from build123d import *

# Parameters (mm, degrees)
CROQUIS1_W              = 10
CROQUIS1_H              = 60
CROQUIS1_R              = 2.5
SALIENTE_EXTRUIR1_DEPTH = 1.5
CROQUIS2_W              = 3
CROQUIS2_H              = 60
SALIENTE_EXTRUIR2_DEPTH = 12
CROQUIS4_R              = 32
CORTAR_EXTRUIR2_DEPTH   = 34.320414163
SKETCH1_W               = 13
SKETCH1_H               = 10
BOSS_EXTRUDE1_DEPTH     = 60
SKETCH2_R               = 2.5
CUT_EXTRUDE1_DEPTH      = 34.109666262
SKETCH3_W               = 10
SKETCH3_H               = 8.5
CUT_EXTRUDE2_DEPTH      = 62.613716005
SKETCH4_R               = 2
CUT_EXTRUDE3_DEPTH      = 34.648922717


with BuildPart() as part:
    # Croquis1 → Saliente-Extruir1 (new body)
    with BuildSketch(Plane(origin=(0, 0, 0), x_dir=(1, 0, 0), z_dir=(0, 1, 0))):
        Rectangle(CROQUIS1_W, CROQUIS1_H)
        with Locations(Location((0, 22.5, 0), (0, 0, 270))):
            Circle(CROQUIS1_R, mode=Mode.SUBTRACT)
        with Locations(Location((0, -22.5, 0), (0, 0, 270))):
            Circle(CROQUIS1_R, mode=Mode.SUBTRACT)
    extrude(amount=SALIENTE_EXTRUIR1_DEPTH)

    # Croquis2 → Saliente-Extruir2 (add)
    with BuildSketch(Plane(origin=(0, 1.5, 0), x_dir=(1, 0, 0), z_dir=(0, 1, 0))):
        with Locations((6.5, 0)):
            Rectangle(CROQUIS2_W, CROQUIS2_H)
    extrude(amount=-SALIENTE_EXTRUIR2_DEPTH)

    # Croquis4 → Cortar-Extruir2 (cut, through all)
    with BuildSketch(Plane.ZY.offset(-5)):
        with Locations((0, -38.5)):
            Circle(CROQUIS4_R)
    extrude(amount=-CORTAR_EXTRUIR2_DEPTH, mode=Mode.SUBTRACT)

    # Sketch1 → Boss-Extrude1 (add)
    with BuildSketch(Plane(origin=(0, 0, -30), x_dir=(-1, 0, 0), z_dir=(0, 0, -1))):
        with Locations((-1.5, 6.5)):
            Rectangle(SKETCH1_W, SKETCH1_H)
    extrude(amount=-BOSS_EXTRUDE1_DEPTH)

    # Sketch2 → Cut-Extrude1 (cut, through all)
    with BuildSketch(Plane.XZ):
        with Locations(Location((0, -22.5, 0), (0, 0, 270))):
            Circle(SKETCH2_R)
        with Locations(Location((0, 22.5, 0), (0, 0, 270))):
            Circle(SKETCH2_R)
    extrude(amount=-CUT_EXTRUDE1_DEPTH, mode=Mode.SUBTRACT)

    # Sketch3 → Cut-Extrude2 (cut, through all)
    with BuildSketch(Plane(origin=(0, 0, -30), x_dir=(-1, 0, 0), z_dir=(0, 0, -1))):
        with Locations((0, 4.25)):
            Rectangle(SKETCH3_W, SKETCH3_H)
    extrude(amount=-CUT_EXTRUDE2_DEPTH, mode=Mode.SUBTRACT)

    # Sketch4 → Cut-Extrude3 (cut, through all)
    with BuildSketch(Plane.ZY.offset(-5)):
        with Locations((-23.57, -4.93)):
            Circle(SKETCH4_R)
    cut_extrude3 = extrude(amount=-CUT_EXTRUDE3_DEPTH, mode=Mode.SUBTRACT)

    # Mirror1: Cut-Extrude3 across plane
    add(cut_extrude3.mirror(Plane.XY), mode=Mode.SUBTRACT)


solid = part.part
CAD build for the part. Positions are in the model's coordinates, mm. A direction names the side the tool comes from. Coordinates: 2 decimals unless noted, no trailing zeros. Loops run counter-clockwise (first coordinate to the right, second up) from the corner with the lowest first, then second, coordinate; pieces in that order, holes last. Notation, with made-up numbers: (-16, -29.75) - (-12, -29.75) arc R23 cw to (-12, 1.25) - close; hole circle Ø4 at (53, 6). An arc over 180 degrees is marked (long way). Use one line per item in the form item = value. Start each with the question number.
1) Two-plate mould, pull along X, no slides. Class faces 1 (the face through (0, 10, 25)), 2 (the face through (0, 8.5, 0)), 3 (the face through (-5, 10, 0)), 4 (the face through (0, 10, -20)): +X half, -X half, draft (parallel to the pull), parting line (faces both ways), or undercut.
2) Flat gauge pins, fed straight in: pin 1 (3 mm diameter, centred on x = 0, z = 22.5, fed in from +Y); pin 2 (5 mm diameter, centred on x = 0.5, z = -13.5, fed in from -Y); pin 3 (2 mm diameter, centred on y = 4.5, z = -14.5, fed in from -X). Where does each tip first touch, or does it go through?
3) Band-saw the part on B-B (z = -21). Give the cut face in (x, y), and give its area (3 significant figures).
4) Band-saw the part on C-C (x = 1.75). Give the cut face in (y, z), and give its area (3 significant figures).
5) Band-saw the part on D-D (y = 9.5). Give the cut face in (x, z).
6) Drill centre lines: L1, parallel to X at y = 10.75, z = 22.5; L2, parallel to X at y = -6, z = 1; L3, parallel to Y at x = 1.25, z = 8. Where is each one in solid material? Low to high. Write a range as from..to.
7) Band-saw the part on A-A (y = -4.93). Give the cut face in (x, z).
8) Tool access for faces 5 (the face through (5.4, 3, 30)), 6 (the face through (5, -1, 0)): list every direction of +Z, -Z, +X, -X, +Y, -Y with a clear straight run to the whole face (end or side of a thin tool).
Check values:
q1.face_1 = undercut
q1.face_2 = draft
q1.face_3 = -X half
q1.face_4 = undercut
q2.pin_1 = through
q2.pin_2 = 8.5
q2.pin_3 = 5
q3.outline = (-5, 8.5) - (-2, 8.5) - (-2, 11.5) - (-5, 11.5) - close; (2, 8.5) - (5, 8.5) - (5, -10.5) - (8, -10.5) - (8, 11.5) - (2, 11.5) - close
q3.area = 84.0 mm2
q4.outline = (8.5, -30) - (11.5, -30) - (11.5, -24.29) - (8.5, -24.29) - close; (8.5, -20.71) - (11.5, -20.71) - (11.5, 20.71) - (8.5, 20.71) - close; (8.5, 24.29) - (11.5, 24.29) - (11.5, 30) - (8.5, 30) - close
q4.area = 159 mm2
q5.outline = (-5, -30) - (8, -30) - (8, 30) - (-5, 30) - close; hole circle Ø5 at (0, -22.5); hole circle Ø5 at (0, 22.5)
q6.L1 = -5..-2.5, 2.5..8
q6.L2 = 5..8
q6.L3 = 8.5..11.5
q7.outline = (5, -30) - (8, -30) - (8, -25.57) - (5, -25.57) - close; (5, -21.57) - (8, -21.57) - (8, 21.57) - (5, 21.57) - close; (5, 25.57) - (8, 25.57) - (8, 30) - (5, 30) - close
q8.face_5 = +Z, +X, -X, +Y, -Y
q8.face_6 = +Z, -Z, -X, -Y
